```python
from build123d import *

# Parameters (mm, degrees)
ESQUISSE1_R             = 11
BOSS_EXTRU_1_DEPTH      = 6.35
ENL_V_MAT_EXTRU_1_DEPTH = 135.686014493
ESQUISSE4_R             = 4
ENL_V_MAT_EXTRU_2_DEPTH = 135.686014493
ESQUISSE5_R             = 11
ENL_V_MAT_EXTRU_3_DEPTH = 135.686014493


with BuildPart() as part:
    # Esquisse1 → Boss.-Extru.1 (new body)
    with BuildSketch(Plane(origin=(0, 0, 0), x_dir=(1, 0, 0), z_dir=(0, 1, 0))):
        with BuildLine():
            Line((-96.654639651, 52.506938663), (-21.654639651, -77.493061337))
            ThreePointArc((-21.654639651, -77.493061337), (0, -90), (21.654639651, -77.493061337))
            Line((21.654639651, -77.493061337), (96.654639651, 52.506938663))
            ThreePointArc((96.654639651, 52.506938663), (96.648631983, 77.50346885), (75, 90))
            Line((75, 90), (-75, 90))
            ThreePointArc((-75, 90), (-96.648631983, 77.50346885), (-96.654639651, 52.506938663))
        make_face()
        with Locations(Location((0, 65, 0), (0, 0, 270))):
            Circle(ESQUISSE1_R, mode=Mode.SUBTRACT)
    extrude(amount=BOSS_EXTRU_1_DEPTH)

    # Esquisse3 → Enlèv. mat.-Extru.1 (cut, through all)
    with BuildSketch(Plane.XZ):
        Polygon((-79.5033321, -82), (-77.25166605, -85.9), (-72.74833395, -85.9), (-70.4966679, -82), (-72.74833395, -78.1), (-77.25166605, -78.1), align=None)
        Polygon((-94.225763964, -56.5), (-91.974097914, -60.4), (-87.470765814, -60.4), (-85.219099765, -56.5), (-87.470765814, -52.6), (-91.974097914, -52.6), align=None)
        Polygon((-64.780900235, -56.5), (-62.529234186, -60.4), (-58.025902086, -60.4), (-55.774236036, -56.5), (-58.025902086, -52.6), (-62.529234186, -52.6), align=None)
        Polygon((55.775701891, -56.499154304), (58.02736794, -60.399154304), (62.53070004, -60.399154304), (64.78236609, -56.499154304), (62.53070004, -52.599154304), (58.02736794, -52.599154304), align=None)
        Polygon((70.498133755, -81.999154304), (72.749799805, -85.899154304), (77.253131904, -85.899154304), (79.504797954, -81.999154304), (77.253131904, -78.099154304), (72.749799805, -78.099154304), align=None)
        Polygon((85.220565619, -56.499154304), (87.472231669, -60.399154304), (91.975563769, -60.399154304), (94.227229819, -56.499154304), (91.975563769, -52.599154304), (87.472231669, -52.599154304), align=None)
        Polygon((-4.5033321, 82), (-2.25166605, 78.1), (2.25166605, 78.1), (4.5033321, 82), (2.25166605, 85.9), (-2.25166605, 85.9), align=None)
        Polygon((10.219099765, 56.5), (12.470765814, 52.6), (16.974097914, 52.6), (19.225763964, 56.5), (16.974097914, 60.4), (12.470765814, 60.4), align=None)
        Polygon((-19.225763964, 56.5), (-16.974097914, 52.6), (-12.470765814, 52.6), (-10.219099765, 56.5), (-12.470765814, 60.4), (-16.974097914, 60.4), align=None)
    extrude(amount=-ENL_V_MAT_EXTRU_1_DEPTH, mode=Mode.SUBTRACT)

    # Esquisse4 → Enlèv. mat.-Extru.2 (cut, through all)
    with BuildSketch(Plane(origin=(0, 6.35, 0), x_dir=(1, 0, 0), z_dir=(0, 1, 0))):
        with Locations(Location((0.000849353, 10.324999995, 0), (0, 0, 270))):
            Circle(ESQUISSE4_R)
    extrude(amount=-ENL_V_MAT_EXTRU_2_DEPTH, mode=Mode.SUBTRACT)

    # Esquisse5 → Enlèv. mat.-Extru.3 (cut, through all)
    with BuildSketch(Plane(origin=(0, 6.35, 0), x_dir=(1, 0, 0), z_dir=(0, 1, 0))):
        with Locations(Location((0, -21, 0), (0, 0, 270))):
            Circle(ESQUISSE5_R)
    extrude(amount=-ENL_V_MAT_EXTRU_3_DEPTH, mode=Mode.SUBTRACT)


solid = part.part
```
The model under review builds one solid part; all positions refer to its coordinate system, in mm. A direction names the side the tool comes from. Coordinates: 2 decimals unless noted, no trailing zeros. Write each loop counter-clockwise with the first axis right and the second up, starting at its lowest first coordinate (ties: lowest second). Pieces come first, ordered by that corner, then holes. Notation, with made-up numbers: (59, -2) -> (88, -2) arc R10 ccw to (88, 10) -> close; hole circle Ø3 at (-8.75, 16). An arc over 180 degrees is marked (long way). One line per item, written item: value. Start each with the question number.
Q1. Add section B-B, the plane x = -7. Give the boundary of the cut face in (y, z), then the cut area to 3 significant figures.
Q2. The part is to be moulded in two halves that separate along Z. For faces 1 (the face through (-15, 3, 52.6)), 2 (the face through (0, 3, 90)), 3 (the face through (-75, 3, -85.9)), 4 (the face through (-96.463, 3.131, -77.819)), say which applies: +Z half, -Z half, draft (parallel to the pull), parting line (faces both ways), or undercut.
Q3. Add section D-D, the plane z = 21. Give the boundary of the cut face in (x, y), then the cut area to 3 significant figures.
Q4. Clearance check with flat-ended pins moving along their axes: P1, Ø1, axis at y = 3, z = -59, coming from the +X side; P2, Ø3.5, axis at x = -75.5, y = 3.5, coming from the +Z side; P3, Ø1.4, axis at x = 61.5, y = 2.5, coming from the +Z side. State where each tip first meets the part, or that it passes through.
Q5. Add section C-C, the plane y = 3. Count the separate pieces of the cut face and the enclosed holes in it, then the cut area to 3 significant figures.
Q6. To check wall thickness, follow probe 1 along X at (y, z) = (4.75, -65); probe 2 along X at (y, z) = (3.5, 13.5); probe 3 along Z at (x, y) = (-71, 0.5). State the ranges of each line that lie inside material, in increasing order.
Q7. Add section A-A, the plane z = -65. Give the boundary of the cut face in (x, y).
Q8. For faces 5 (the face through (-1, 6.35, -21)), 6 (the face through (60, 3, -52.599)), list the 3-axis set-ups (+Z, -Z, +X, -X, +Y, -Y) from which the entire face can be reached by the end or side of a thin tool; tool diameter is ignored.
Response:
1. outline: (0, -90) -> (6.35, -90) -> (6.35, -73.49) -> (0, -73.49) -> close; (0, -56.51) -> (6.35, -56.51) -> (6.35, 12.51) -> (0, 12.51) -> close; (0, 29.49) -> (6.35, 29.49) -> (6.35, 89) -> (0, 89) -> close
1. area: 921 mm²
2. face 1: undercut
2. face 2: +Z half
2. face 3: undercut
2. face 4: parting line
3. outline: (-54.25, 0) -> (-11, 0) -> (-11, 6.35) -> (-54.25, 6.35) -> close; (11, 0) -> (54.25, 0) -> (54.25, 6.35) -> (11, 6.35) -> close
3. area: 549 mm²
4. P1: x = 99.39
4. P2: z = -12.81
4. P3: z = 9.64
5. separate pieces: 1
5. enclosed holes: 12
5. area: 21,700 mm²
6. probe 1: -100 to -11, 11 to 100
6. probe 2: -58.57 to -8.05, 8.05 to 58.57
6. probe 3: -90 to -82.87, -81.13 to -8.04
7. outline: (-100, 0) -> (-11, 0) -> (-11, 6.35) -> (-100, 6.35) -> close; (11, 0) -> (100, 0) -> (100, 6.35) -> (11, 6.35) -> close
8. face 5: +Z, -Z, +X, -X, +Y
8. face 6: +Y, -Y
